Source: CAD feature listing. Evaluate the final solid. Frame: model axes, mm. Face numbers are marked on the shaded views. A direction names the side the tool comes from. Coordinates: 2 decimals unless noted, no trailing zeros. Order: outer loops, then holes, each group sorted by start corner. A loop starts at its lowest first (then second) coordinate and runs counter-clockwise, first axis right, second up.
Item 1: Reachability of the marked faces 4, 5 and 6 from +Z, -Z, +X, -X, +Y, -Y: full face, straight path, thin tool, end or side. Return the list, or none.
Item 2: Section D-D on y = 2.5. Return the cut outline in (x, z), then the cut area to 3 significant figures.
Item 3: Mould query, pull axis Y, two halves, no side actions, for the marked faces 1, 2 and 3. Classes: released by +Y, released by -Y, zero draft, split by the parting line, or undercut.
Item 4: Section B-B on x = 10. Return the cut outline in (y, z).
Item 5: Contact query for flat-ended pins moving along their axis: P1, Ø9, axis at x = 9, z = 4.5, coming from the +Y side; P2, Ø14, axis at x = 35, y = 16.5, coming from the -Z side; P3, Ø1.5, axis at y = 21, z = 6, coming from the -X side. Output: stop coordinate, or through.
Item 6: Ray query, line 1 (Z direction, x = 60, y = 4); line 2 (X direction, y = 15, z = 7.6); line 3 (Y direction, x = 35, z = 7.6). Return the intervals inside material, ascending.
Item 7: Section A-A on z = 9. Return the cut outline in (x, y).
Item 8: Section C-C on z = 16.5. Return the cut outline in (x, y).
from build123d import *

# Parameters (mm, degrees)
F0_R     = 6
F1_DEPTH = 18
F2_R     = 6
F3_DEPTH = 6
F4_R     = 3
F5_DEPTH = 25
F6_R     = 6
F7_DEPTH = 6


with BuildPart() as f1:
    # F0 (on Top) → F1 (new body)
    with BuildSketch(Plane.XY):
        Polygon((0, 10), (0, 0), (70, 0), (70, 10), (50, 10), (50, 30), (20, 30), (20, 10), align=None)
        with Locations((35, 15)):
            Circle(F0_R, mode=Mode.SUBTRACT)
    extrude(amount=F1_DEPTH)

    # F2 (on face) → F3 (cut)
    with BuildSketch(Plane.XY.offset(18)):
        Polygon((40.051815, 23.75), (29.948185, 23.75), (24.89637, 15), (29.948185, 6.25), (40.051815, 6.25), (45.10363, 15), align=None)
        with Locations((35, 15)):
            Circle(F2_R, mode=Mode.SUBTRACT)
    extrude(amount=-F3_DEPTH, mode=Mode.SUBTRACT)

    # F4 (on face) → F5 (cut)
    with BuildSketch(Plane(origin=(0, 10, 0), x_dir=(-1, 0, 0), z_dir=(0, 1, 0))):
        with Locations((-60, 9)):
            Circle(F4_R)
        with Locations((-10, 9)):
            Circle(F4_R)
    extrude(amount=-F5_DEPTH, mode=Mode.SUBTRACT)

    # F6 (on face) → F7 (cut)
    with BuildSketch(Plane(origin=(0, 0, 0), x_dir=(1, 0, 0), z_dir=(0, 0, -1))):
        Polygon((29.948185, -23.75), (40.051815, -23.75), (45.10363, -15), (40.051815, -6.25), (29.948185, -6.25), (24.89637, -15), align=None)
        with Locations((35, -15)):
            Circle(F6_R, mode=Mode.SUBTRACT)
    extrude(amount=-F7_DEPTH, mode=Mode.SUBTRACT)


solid = f1.part
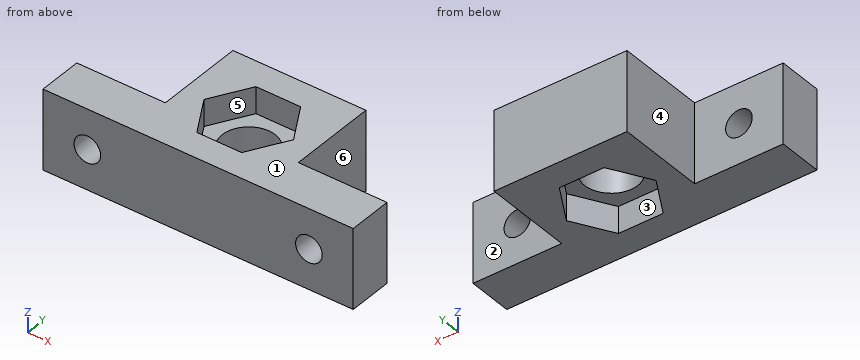
Answer list:
1. face 4: +Z, -Z, -X, +Y
1. face 5: +Z
1. face 6: +Z, -Z, +X, +Y
2. outline: (0, 0) - (70, 0) - (70, 18) - (0, 18) - close; hole circle Ø6 at (10, 9); hole circle Ø6 at (60, 9)
2. area: 1,200 mm2
3. face 1: zero draft
3. face 2: released by +Y
3. face 3: undercut
4. outline: (0, 0) - (10, 0) - (10, 6) - (0, 6) - close; (0, 12) - (10, 12) - (10, 18) - (0, 18) - close
5. P1: stops at y = 10
5. P2: stops at z = 6
5. P3: stops at x = 20
6. line 1: z = 0 to 6, 12 to 18
6. line 2: x = 20 to 29, 41 to 50
6. line 3: y = 0 to 9, 21 to 30
7. outline: (0, 0) - (7, 0) - (7, 10) - (0, 10) - close; (13, 0) - (57, 0) - (57, 10) - (50, 10) - (50, 30) - (20, 30) - (20, 10) - (13, 10) - close; (63, 0) - (70, 0) - (70, 10) - (63, 10) - close; hole circle Ø12 at (35, 15)
8. outline: (0, 0) - (70, 0) - (70, 10) - (50, 10) - (50, 30) - (20, 30) - (20, 10) - (0, 10) - close; hole (24.9, 15) - (29.95, 6.25) - (40.05, 6.25) - (45.1, 15) - (40.05, 23.75) - (29.95, 23.75) - close
